The model under review builds one solid part; all positions refer to its coordinate system, in mm. A direction names the side the tool comes from. Round coordinates to 2 decimals unless told otherwise and drop trailing zeros. Order: outer loops, then holes, each group sorted by start corner. A loop starts at its lowest first (then second) coordinate and runs counter-clockwise, first axis right, second up.
1) To check wall thickness, follow L1, parallel to X at y = -0.6, z = 0 (3 decimals); L2, parallel to X at y = 3, z = 3. State the ranges of each line that lie inside material, in increasing order.
2) Machinability: for faces 1 (the face through (-21.15, 17, 4)), 2 (the face through (31, 1.25, 0)), 3 (the face through (-22.95, 18, 5)), which of the approach directions +Z, -Z, +X, -X, +Y, -Y give a long, thin tool a straight path to every point of the face, cutting with its end or side? Answer none if there is none.
3) Consider section A-A (x = 0). Give the boundary of the cut face in (y, z), then the cut area to 3 significant figures.
4) Mouldability with a two-part tool opening along Z and no side actions: class faces 4 (the face through (30.48, 0.02, -19.1)), 5 (the face through (-28.52, -0.82, -0.22)), 6 (the face through (21.15, 17, 4)) as pulls with the +Z half, pulls with the -Z half, needs draft (parallel to the pull), parting line crosses it, or undercut.
5) Clearance check with flat-ended pins moving along their axes: P1, Ø1.5, axis at x = 23, y = 34, coming from the -Z side; P2, Ø4, axis at y = 17.5, z = 4.5, coming from the -X side; P3, Ø4, axis at x = -15.975, y = 38.475, coming from the +Z side; P4, Ø1.5, axis at y = 7, z = 13.5, coming from the +X side. State where each tip first meets the part, or that it passes through.
6) Consider section D-D (z = -10). Give the boundary of the cut face in (x, y) (3 decimals), then the cut area to 3 significant figures.
7) Consider section C-C (y = 22.5). Give the boundary of the cut face in (x, z), then the cut area to 3 significant figures.
8) Consider section B-B (z = -15.5). Give the boundary of the cut face in (x, y) (3 decimals), then the cut area to 3 significant figures.
from build123d import *
from OCP.BRepFilletAPI import BRepFilletAPI_MakeChamfer

# Parameters (mm, degrees)
RESSALTO_EXTRUS_O1_DEPTH            = 1.25
ESBO_O2_W                           = 45.9
ESBO_O2_H                           = 40
ESBO_O2_W_2                         = 42.3
ESBO_O2_H_2                         = 36.4
RESSALTO_EXTRUS_O2_DEPTH            = 42
CORTE_EXTRUS_O1_DEPTH               = 58.030208881
CORTE_EXTRUS_O1_DEPTH_BACK          = 58.030208881
ESBO_O5_R                           = 11.25
CORTE_EXTRUS_O2_DEPTH               = 67.726641793
ESBO_O6_R                           = 1.65
CORTE_EXTRUS_O3_DEPTH               = 67.726641793
ESBO_O7_W                           = 42.3
ESBO_O7_H                           = 1.8
CORTE_EXTRUS_O4_DEPTH               = 57.08816475
ESCAREADO_PARA_SFHCS_M31_AT_2_COUNT = 2
ESCAREADO_PARA_SFHCS_M31_AT_2_PITCH = 15.5
ESCAREADO_PARA_SFHCS_M31_AT_3_COUNT = 2
ESCAREADO_PARA_SFHCS_M31_AT_3_PITCH = 15.5
ESCAREADO_PARA_SFHCS_M31_AT_4_COUNT = 2
ESCAREADO_PARA_SFHCS_M31_AT_4_PITCH = 55.863394992
ESCAREADO_PARA_SFHCS_M31_AT_5_COUNT = 2
ESCAREADO_PARA_SFHCS_M31_AT_5_PITCH = 53.67
ESCAREADO_PARA_SFHCS_M31_AT_6_COUNT = 2
ESCAREADO_PARA_SFHCS_M31_AT_6_PITCH = 55.863394992
CHANFRO1_SIZE                       = 0.5
CHANFRO1_SIZE2                      = 0.866025404
CHANFRO2_SIZE                       = 0.2


with BuildPart() as part:
    # Esboço1 → Ressalto-extrusão1 (new, symmetric)
    with BuildSketch(Plane(origin=(0, 0, 0), x_dir=(1, 0, 0), z_dir=(0, 1, 0))):
        with BuildLine():
            Line((-28.335, -20), (28.335, -20))
            ThreePointArc((28.335, -20), (30.456320344, -19.121320344), (31.335, -17))
            Line((31.335, -17), (31.335, 17))
            ThreePointArc((31.335, 17), (30.456320344, 19.121320344), (28.335, 20))
            Line((28.335, 20), (-28.335, 20))
            ThreePointArc((-28.335, 20), (-30.456320344, 19.121320344), (-31.335, 17))
            Line((-31.335, 17), (-31.335, -17))
            ThreePointArc((-31.335, -17), (-30.456320344, -19.121320344), (-28.335, -20))
        make_face()
    extrude(amount=RESSALTO_EXTRUS_O1_DEPTH, both=True)

    # Esboço2 → Ressalto-extrusão2 (add)
    with BuildSketch(Plane(origin=(0, 1.25, 0), x_dir=(1, 0, 0), z_dir=(0, 1, 0))):
        Rectangle(ESBO_O2_W, ESBO_O2_H)
        Rectangle(ESBO_O2_W_2, ESBO_O2_H_2, mode=Mode.SUBTRACT)
    extrude(amount=RESSALTO_EXTRUS_O2_DEPTH)

    # Esboço4 → Corte-extrusão1 (cut, two sides: drawn at the far end of the back side and taken through both)
    with BuildSketch(Plane(origin=(0, 0, 0), x_dir=(0, 0, -1), z_dir=(1, 0, 0)).offset(-CORTE_EXTRUS_O1_DEPTH_BACK)):
        Polygon((-18.2, 43.25), (20, 1.25), (20, 43.25), align=None)
    extrude(amount=CORTE_EXTRUS_O1_DEPTH + CORTE_EXTRUS_O1_DEPTH_BACK, mode=Mode.SUBTRACT)

    # Esboço5 → Corte-extrusão2 (cut, through all)
    with BuildSketch(Plane.XY.offset(20)):
        with Locations((0, 22.5)):
            Circle(ESBO_O5_R)
    extrude(amount=-CORTE_EXTRUS_O2_DEPTH, mode=Mode.SUBTRACT)

    # Esboço6 → Corte-extrusão3 (cut, through all)
    with BuildSketch(Plane.XY.offset(20)):
        with Locations((-15.975, 38.475)):
            Circle(ESBO_O6_R)
        with Locations((15.975, 38.475)):
            Circle(ESBO_O6_R)
        with Locations((15.975, 6.525)):
            Circle(ESBO_O6_R)
        with Locations((-15.975, 6.525)):
            Circle(ESBO_O6_R)
    extrude(amount=-CORTE_EXTRUS_O3_DEPTH, mode=Mode.SUBTRACT)

    # Esboço7 → Corte-extrusão4 (cut, through all)
    with BuildSketch(Plane(origin=(0, 1.25, 0), x_dir=(1, 0, 0), z_dir=(0, 1, 0))):
        with Locations((0, 19.1)):
            Rectangle(ESBO_O7_W, ESBO_O7_H)
    extrude(amount=CORTE_EXTRUS_O4_DEPTH, mode=Mode.SUBTRACT)

    # Esboço9 → Escareado para SFHCS M31 (revolve, cut)
    with BuildSketch(Plane(origin=(-26.835, 1.25, 0), x_dir=(0, 0, 1), z_dir=(1, 0, 0))):
        Polygon((0, 0), (0, 2.5), (1.7, 2.5), (1.7, 1.66), (3.36, 0), align=None)
    escareado_para_sfhcs_m31 = revolve(axis=Axis((-26.835, 7.6, 0), (0, -1, 0)), mode=Mode.SUBTRACT)

    # Escareado para SFHCS M31 at 2: Escareado para SFHCS M31 ×2
    with Locations(*[(0, 0, i * ESCAREADO_PARA_SFHCS_M31_AT_2_PITCH) for i in range(1, ESCAREADO_PARA_SFHCS_M31_AT_2_COUNT)]):
        add(escareado_para_sfhcs_m31, mode=Mode.SUBTRACT)

    # Escareado para SFHCS M31 at 3: Escareado para SFHCS M31 ×2
    with Locations(*[(0, 0, -i * ESCAREADO_PARA_SFHCS_M31_AT_3_PITCH) for i in range(1, ESCAREADO_PARA_SFHCS_M31_AT_3_COUNT)]):
        add(escareado_para_sfhcs_m31, mode=Mode.SUBTRACT)

    # Escareado para SFHCS M31 at 4: Escareado para SFHCS M31 ×2
    with Locations(*[Vector(0.9607364537719713, 0, -0.2774625495335487) * (i * ESCAREADO_PARA_SFHCS_M31_AT_4_PITCH) for i in range(1, ESCAREADO_PARA_SFHCS_M31_AT_4_COUNT)]):
        add(escareado_para_sfhcs_m31, mode=Mode.SUBTRACT)

    # Escareado para SFHCS M31 at 5: Escareado para SFHCS M31 ×2
    with Locations(*[(i * ESCAREADO_PARA_SFHCS_M31_AT_5_PITCH, 0, 0) for i in range(1, ESCAREADO_PARA_SFHCS_M31_AT_5_COUNT)]):
        add(escareado_para_sfhcs_m31, mode=Mode.SUBTRACT)

    # Escareado para SFHCS M31 at 6: Escareado para SFHCS M31 ×2
    with Locations(*[Vector(0.9607364537719713, 0, 0.2774625495335487) * (i * ESCAREADO_PARA_SFHCS_M31_AT_6_PITCH) for i in range(1, ESCAREADO_PARA_SFHCS_M31_AT_6_COUNT)]):
        add(escareado_para_sfhcs_m31, mode=Mode.SUBTRACT)

    # Chanfro1: one chamfer whose edges measure the first distance from different faces: ONE call of the kernel's chamfer builder (chamfer() names one face for all edges)
    chanfro1_edges_1 = [part.edges().sort_by_distance(p)[0] for p in [
        (-22.95, 1.25, 0),
    ]]
    chanfro1_side_1 = [part.faces().sort_by_distance(p)[0] for p in [
        (-30.167330013, 1.25, 18.832330013),
    ]]
    chanfro1_edges_2 = [part.edges().sort_by_distance(p)[0] for p in [
        (22.95, 1.25, 0),
    ]]
    chanfro1_side_2 = [part.faces().sort_by_distance(p)[0] for p in [
        (23.358694045, 1.25, 0),
    ]]
    chanfro1 = BRepFilletAPI_MakeChamfer(part.part.solid().wrapped)
    for e in chanfro1_edges_1:
        chanfro1.Add(CHANFRO1_SIZE, CHANFRO1_SIZE2, e.wrapped, chanfro1_side_1[0].wrapped)  # the first distance lies on this face
    for e in chanfro1_edges_2:
        chanfro1.Add(CHANFRO1_SIZE, CHANFRO1_SIZE2, e.wrapped, chanfro1_side_2[0].wrapped)  # the first distance lies on this face
    add(Compound.cast(chanfro1.Shape()), mode=Mode.REPLACE)

    # Chanfro2
    chanfro2_edges = [part.edges().sort_by_distance(p)[0] for p in [
        (-11.25, 22.5, 18.2),
        (-11.25, 22.5, 20),
        (-17.625, 6.525, 20),
        (14.325, 6.525, 20),
        (14.325, 38.475, 20),
        (-17.625, 38.475, 20),
    ]]
    chamfer(chanfro2_edges, length=CHANFRO2_SIZE)


solid = part.part
Answer below:
1. L1: x = -31.335 to -28.535, -25.135 to 25.135, 28.535 to 31.335
1. L2: x = -22.95 to -21.15, 21.15 to 22.95
2. face 1: -Z, +Y
2. face 2: +Z, -Z, +X, +Y
2. face 3: +Z, -Z, -X, +Y
3. outline: (-1.25, -20) - (1.25, -20) - (1.25, 18.2) - (11.05, 18.2) - (11.25, 18.4) - (11.25, 19.8) - (11.05, 20) - (-1.25, 20) - close; (33.75, 18.4) - (33.95, 18.2) - (43.25, 18.2) - (43.25, 20) - (33.95, 20) - (33.75, 19.8) - close
3. area: 135 mm2
4. face 4: pulls with the -Z half
4. face 5: undercut
4. face 6: needs draft
5. P1: stops at z = 9.11
5. P2: stops at x = -22.95
5. P3: stops at z = 20
5. P4: stops at x = 22.95
6. outline: (-31.335, -1.25) - (31.335, -1.25) - (31.335, 1.25) - (23.45, 1.25) - (22.95, 2.116) - (22.95, 12.245) - (21.15, 12.245) - (21.15, 1.25) - (-21.15, 1.25) - (-21.15, 12.245) - (-22.95, 12.245) - (-22.95, 2.116) - (-23.45, 1.25) - (-31.335, 1.25) - close
6. area: 197 mm2
7. outline: (-22.95, -0.67) - (-21.15, -0.67) - (-21.15, 18.2) - (-11.45, 18.2) - (-11.25, 18.4) - (-11.25, 19.8) - (-11.45, 20) - (-22.95, 20) - close; (11.25, 18.4) - (11.45, 18.2) - (21.15, 18.2) - (21.15, -0.67) - (22.95, -0.67) - (22.95, 20) - (11.45, 20) - (11.25, 19.8) - close
7. area: 110 mm2
8. outline: (-31.335, -1.25) - (-28.535, -1.25) - (-28.535, -0.41) - (-30.195, 1.25) - (-31.335, 1.25) - close; (-25.135, -1.25) - (25.135, -1.25) - (25.135, -0.41) - (23.475, 1.25) - (23.45, 1.25) - (22.95, 2.116) - (22.95, 6.198) - (21.15, 6.198) - (21.15, 1.25) - (-21.15, 1.25) - (-21.15, 6.198) - (-22.95, 6.198) - (-22.95, 2.116) - (-23.45, 1.25) - (-23.475, 1.25) - (-25.135, -0.41) - close; (28.535, -1.25) - (31.335, -1.25) - (31.335, 1.25) - (30.195, 1.25) - (28.535, -0.41) - close
8. area: 152 mm2
